Source: three-view drawing plus pictorial views. Frame: mm from the lowest corner of the part. A direction names the side the tool comes from. Give positions to 0.01 mm unless a question says otherwise; leave off trailing zeros. Loops run counter-clockwise (first coordinate to the right, second up) from the corner with the lowest first, then second, coordinate; pieces in that order, holes last. Notation, with made-up numbers: M 75,31.25 L 103,31.25 A28 ccw 103,70.25 Z; hole C -27,38 d2. An arc over 180 degrees is marked long. One line per item, written item: value. Start each with the question number.
(1) Access query for the marked faces 1, 2 and 3. Directions: +Z, -Z, +X, -X, +Y, -Y. A direction counts if a zero-diameter tool reaches every point of the face in a straight line with its end or side. Return the directions, or none.
(2) Section A-A on x = 76.2. Output: boundary loops of the cut face in (y, z).
(3) Section D-D on x = 124.5. Output: boundary loops of the cut face in (y, z), plus the area to 3 significant figures.
(4) Section B-B on z = 76.2. Output: boundary loops of the cut face in (x, y), plus the area to 3 significant figures.
(5) Ray query, line 1 along Z through (x, y) = (76, 23); line 2 along X through (y, z) = (71, 76). Return the intervals inside material, ascending. Write a range as from..to.
(6) Pin query (flat end, axial travel): P1, Ø5, axis at x = 18.5, z = 61.5, coming from the -Y side; P2, Ø1, axis at x = 79, y = 19.5, coming from the +Z side; P3, Ø1.5, axis at y = 28, z = 61.5, coming from the +X side. Return the tip coordinate at first contact, or that it passes through.
(7) Section C-C on y = 47.5. Output: boundary loops of the cut face in (x, z), plus the area to 3 significant figures.
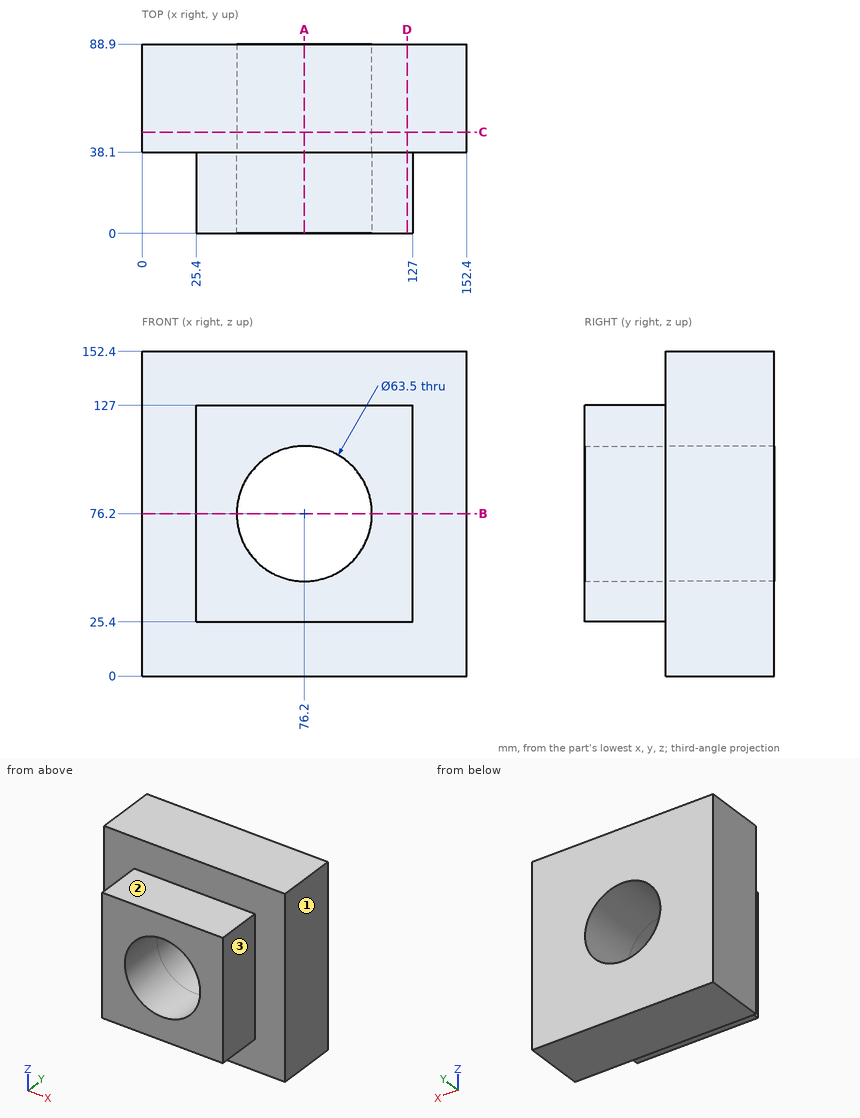
Output values:
1. face 1: +Z, -Z, +X, +Y, -Y
1. face 2: +Z, +X, -X, -Y
1. face 3: +Z, -Z, +X, -Y
2. outline: M 0,25.4 L 38.1,25.4 L 38.1,0 L 88.9,0 L 88.9,44.45 L 0,44.45 Z; M 0,107.95 L 88.9,107.95 L 88.9,152.4 L 38.1,152.4 L 38.1,127 L 0,127 Z
3. outline: M 0,25.4 L 38.1,25.4 L 38.1,0 L 88.9,0 L 88.9,152.4 L 38.1,152.4 L 38.1,127 L 0,127 Z
3. area: 11,600 mm²
4. outline: M 0,38.1 L 25.4,38.1 L 25.4,0 L 44.45,0 L 44.45,88.9 L 0,88.9 Z; M 107.95,0 L 127,0 L 127,38.1 L 152.4,38.1 L 152.4,88.9 L 107.95,88.9 Z
4. area: 5,970 mm²
5. line 1: z = 25.4..44.45, 107.95..127
5. line 2: x = 0..44.45, 107.95..152.4
6. P1: stops at y = 38.1
6. P2: stops at z = 127
6. P3: stops at x = 127
7. outline: M 0,0 L 152.4,0 L 152.4,152.4 L 0,152.4 Z; hole C 76.2,76.2 d63.5
7. area: 20,100 mm²
